CAD build for the part. Positions are in the model's coordinates, mm. A direction names the side the tool comes from. Round coordinates to 2 decimals unless told otherwise and drop trailing zeros. Loops run counter-clockwise (first coordinate to the right, second up) from the corner with the lowest first, then second, coordinate; pieces in that order, holes last. Notation, with made-up numbers: M 11,85.25 L 56,85.25 A17 ccw 56,101.25 Z; hole C -6,15 d2. An arc over 180 degrees is marked long. Use one line per item in the form item = value.
from build123d import *

# Parameters (mm, degrees)
F0_W      = 127
F0_H      = 50.8
F1_DEPTH  = 38.1
F3_DEPTH  = 38.1
F4_R      = 6.35
F5_DEPTH  = 25.4
F6_R      = 6.35
F7_DEPTH  = 25.4
F8_W      = 25.4
F8_H      = 38.202004
F9_DEPTH  = 38.1
F11_DEPTH = 25.4


with BuildPart() as f1:
    # F0 (on Front) → F1 (new body)
    with BuildSketch(Plane.XZ):
        with Locations((-2.091765, 1.867647)):
            Rectangle(F0_W, F0_H)
    extrude(amount=F1_DEPTH)

    # F2 (on face) → F3 (cut)
    with BuildSketch(Plane.XZ.offset(38.1)):
        Polygon((36.008235, 1.867647), (61.408235, 1.867647), (61.408235, 27.267647), (23.308235, 27.267647), align=None)
        Polygon((-65.591765, 27.267647), (-65.591765, 1.867647), (-40.191765, 1.867647), (-27.491765, 27.267647), align=None)
    extrude(amount=-F3_DEPTH, mode=Mode.SUBTRACT)

    # F4 (on face) → F5 (cut)
    with BuildSketch(Plane.XY.offset(1.867647)):
        with Locations((48.708235, -19.05)):
            Circle(F4_R)
    extrude(amount=-F5_DEPTH, mode=Mode.SUBTRACT)

    # F6 (on face) → F7 (cut)
    with BuildSketch(Plane.XY.offset(1.867647)):
        with Locations((-52.891765, -19.05)):
            Circle(F6_R)
    extrude(amount=-F7_DEPTH, mode=Mode.SUBTRACT)

    # F8 (on face) → F9 (cut)
    with BuildSketch(Plane.XY.offset(27.267647)):
        with Locations((-2.091765, -18.998998)):
            Rectangle(F8_W, F8_H)
    extrude(amount=-F9_DEPTH, mode=Mode.SUBTRACT)

    # F10 (on face) → F11 (join)
    with BuildSketch(Plane.YZ.offset(-14.791765)):
        Polygon((-14.572936, 27.267647), (-36.569981, -10.832353), (0, -10.832353), (0, 27.267647), align=None)
    extrude(amount=F11_DEPTH)


solid = f1.part
1. Drop flat-ended pins along their axis: P1, Ø1.2, axis at x = -5, y = -37.5, coming from the +Z side; P2, Ø7.5, axis at x = 52.5, y = -24.5, coming from the +Z side; P3, Ø4, axis at y = -15.5, z = 18.5, coming from the -X side; P4, Ø7.5, axis at x = -52.89, y = -19.05, coming from the +Z side. Give the stop position or say it passes through.
Completed:
P1 = -10.83
P2 = 1.87
P3 = -32.88
P4 = through
2. Probe line 1 along X through (y, z) = (-19, -11); line 2 along Z through (x, y) = (-60, -7); line 3 along X through (y, z) = (-23.5, -7.5). List the from-to ranges inside material, lowest first. Write a range as from..to.
Completed:
line_1 = -65.59..-59.24, -46.54..42.36, 55.06..61.41
line_2 = -23.53..1.87
line_3 = -65.59..-57.42, -48.36..44.18, 53.24..61.41
3. Tool access for faces 4 (the face through (10.608, -29, 13)), 5 (the face through (54, -24, 1.868)), 6 (the face through (-59, -24, 1.868)): list every direction of +Z, -Z, +X, -X, +Y, -Y with a clear straight run to the whole face (end or side of a thin tool).
Completed:
face_4 = +Z, -Y
face_5 = +Z, +X, +Y, -Y
face_6 = +Z, -X, +Y, -Y
4. Cut at A-A on y = -22. Write the cut outline in (x, z).
Completed:
outline = M -65.59,-23.53 L -58.51,-23.53 L -58.51,1.87 L -65.59,1.87 Z; M -47.27,-23.53 L 43.09,-23.53 L 43.09,1.87 L 36.01,1.87 L 23.31,27.27 L 10.61,27.27 L 10.61,14.4 L -14.79,14.4 L -14.79,27.27 L -27.49,27.27 L -40.19,1.87 L -47.27,1.87 Z; M 54.33,-23.53 L 61.41,-23.53 L 61.41,1.87 L 54.33,1.87 Z
5. Cut at B-B on x = -58. Write the cut outline in (y, z).
Completed:
outline = M -38.1,-23.53 L -22.82,-23.53 L -22.82,1.87 L -38.1,1.87 Z; M -15.28,-23.53 L 0,-23.53 L 0,1.87 L -15.28,1.87 Z
6. Pull direction Y, two halves, no side cores. Call faces 1 (the face through (-2.27, -25.42, 8.48)), 2 (the face through (-14.792, -29, 13)), 3 (the face through (-47.026, -21.482, -10.655)): +Y half, -Y half, draft (parallel to the pull), parting line (faces both ways), or undercut.
Completed:
face_1 = -Y half
face_2 = draft
face_3 = undercut
7. Cut at C-C on z = 3.5. Write the cut outline in (x, y).
Completed:
outline = M -39.38,-38.1 L -14.79,-38.1 L -14.79,-28.3 L 10.61,-28.3 L 10.61,-38.1 L 35.19,-38.1 L 35.19,0 L -39.38,0 Z
8. Cut at D-D on y = -32. Write the cut outline in (x, z).
Completed:
outline = M -65.59,-23.53 L 61.41,-23.53 L 61.41,1.87 L 36.01,1.87 L 23.31,27.27 L 10.61,27.27 L 10.61,-2.92 L -14.79,-2.92 L -14.79,27.27 L -27.49,27.27 L -40.19,1.87 L -65.59,1.87 Z
